from build123d import *

# Parameters (mm, degrees)
BOSS_EXTRUDE1_DEPTH = 17.5
BOSS_EXTRUDE2_START = -1.75
BOSS_EXTRUDE2_DEPTH = 0.5
CHAMFER1_SIZE       = 0.2


with BuildPart() as part:
    # Sketch1 → Boss-Extrude1 (new, symmetric)
    with BuildSketch(Plane(origin=(0, 0, 0), x_dir=(1, 0, 0), z_dir=(0, 1, 0))):
        with BuildLine():
            Line((-1.25, -3), (1.25, -3))
            ThreePointArc((1.25, -3), (0, 3.25), (-1.25, -3))
        make_face()
    extrude(amount=BOSS_EXTRUDE1_DEPTH, both=True)

    # Sketch2 → Boss-Extrude2 (add)
    with BuildSketch(Plane.XZ.offset(17.5).offset(BOSS_EXTRUDE2_START)):
        with BuildLine():
            Line((-1.25, 3), (-1.6, 3))
            ThreePointArc((-1.6, 3), (0, -3.4), (1.6, 3))
            Line((1.6, 3), (1.25, 3))
            ThreePointArc((1.25, 3), (0, -3.25), (-1.25, 3))
        make_face()
    extrude(amount=BOSS_EXTRUDE2_DEPTH)

    # Chamfer1
    # the kernel refuses this chamfer: 0.2 mm, written as the material it takes off along each edge
    with BuildSketch(Plane(origin=(0, -15.75, 0), x_dir=(-0.3315887986155938, 0, 0.9434240131736458), z_dir=(0.9434240131736458, 0, 0.3315887986155938))) as chamfer1_piece_1_section:
        Polygon((3.4, CHAMFER1_SIZE), (3.4 - CHAMFER1_SIZE, 0), (3.4, 0), align=None)
    chamfer1_piece_1 = revolve(axis=Axis((0, -15.75, 0), (0, -1, 0)), revolution_arc=321.269525005, mode=Mode.PRIVATE)
    chamfer1_piece_1 = chamfer1_piece_1 - Plane(origin=(0, -15.75, 0), x_dir=(0.38461538461538497, 0, 0.923076923076923), z_dir=(0, 1, 0)) * Cylinder(3.25, 14, mode=Mode.PRIVATE)
    add(chamfer1_piece_1, mode=Mode.SUBTRACT)

    # Chamfer2: read off the stored shape, not the designer's step
    # Chamfer2 outline → Chamfer2 (revolve, cut)
    with BuildSketch(Plane.XY):
        Polygon((3.25, 17.5), (2.75, 17.5), (3.25, 17), align=None)
    revolve(axis=Axis((0, 0, 0), (0, 1, 0)), mode=Mode.SUBTRACT)


solid = part.part
Build history of the part. All positions in model axes, mm. A direction names the side the tool comes from. Give positions to 0.01 mm unless a question says otherwise; leave off trailing zeros. Order: outer loops, then holes, each group sorted by start corner. A loop starts at its lowest first (then second) coordinate and runs counter-clockwise, first axis right, second up. Notation, with made-up numbers: M -14.5,58.5 L 18.5,58.5 A32 ccw 18.5,90.5 Z; hole C 12.25,66 d11. An arc over 180 degrees is marked long. Put each result on its own line as item: value.
Item 1: Two-plate mould, pull along X, no slides. Class faces 1 (the cylindrical face through (0.125, 0.83, -3.248)), 2 (the flat face through (0, -17.5, 0)): +X half, -X half, draft (parallel to the pull), parting line (faces both ways), or undercut.
From the geometry:
face 1: parting line
face 2: draft
Item 2: Flat gauge pins, fed straight in: pin 1 Ø1.5 at (y, z) = (-10.5, 0) entering from +X; pin 2 Ø1 at (y, z) = (-14, -1.5) entering from +X; pin 3 Ø1 at (y, z) = (-1.5, 0.5) entering from -X. Where does each tip first touch, or does it go through?
From the geometry:
pin 1: stops at x = 3.25
pin 2: stops at x = 3.09
pin 3: stops at x = -3.25
Item 3: 3-axis set-ups, long thin cutter, end or side, ignore diameter. For faces 3 (the cylindrical face through (0.125, -16.866, -3.248)), 4 (the cylindrical face through (-0.1, -16.1, -3.4)): which of +Z, -Z, +X, -X, +Y, -Y reach the whole face in a straight line?
From the geometry:
face 3: -Y
face 4: +Y, -Y
Item 4: Slice it at B-B, the plane z = 0. Write the cut outline in (x, y).
From the geometry:
outline: M -3.4,-16.25 L -3.25,-16.25 L -3.25,-17.5 L 3.25,-17.5 L 3.25,-16.25 L 3.4,-16.25 L 3.4,-15.95 L 3.25,-15.8 L 3.25,17 L 2.75,17.5 L -2.75,17.5 L -3.25,17 L -3.25,-15.8 L -3.4,-15.95 Z
Item 5: Slice it at C-C, the plane y = 1. Write the cut outline in (x, z).
From the geometry:
outline: M -1.25,3 A3.25 ccw long 1.25,3 Z
Item 6: Slice it at A-A, the plane x = 0. Write the cut outline in (y, z), plus the area to 3 significant figures.
From the geometry:
outline: M -17.5,-3.25 L -16.25,-3.25 L -16.25,-3.4 L -15.95,-3.4 L -15.8,-3.25 L 17,-3.25 L 17.5,-2.75 L 17.5,2.75 L 17.25,3 L -17.5,3 Z
area: 219 mm2
Item 7: Probe line 1 (X direction, y = 14, z = -1); line 2 (Z direction, x = 0.75, y = 6.5); line 3 (X direction, y = -9, z = 1.25). List the from-to ranges inside material, lowest first. Write a range as [from, to].
From the geometry:
line 1: x = [-3.09, 3.09]
line 2: z = [-3.16, 3]
line 3: x = [-3, 3]
